from build123d import *
from build123d.topology import SkipClean

# Parameters (mm, degrees)
SKETCH1_R           = 8.89
BOSS_EXTRUDE1_DEPTH = 31.75
SKETCH2_R           = 3.302
BOSS_EXTRUDE2_DEPTH = 4.572
SKETCH3_R           = 11.938
BOSS_EXTRUDE3_DEPTH = 1.524


with BuildPart() as part:
    # Sketch1 → Boss-Extrude1 (new body)
    with BuildSketch(Plane(origin=(0, 0, 0), x_dir=(1, 0, 0), z_dir=(0, 1, 0))):
        with Locations(Location((0, 0, 0), (0, 0, 270))):
            Circle(SKETCH1_R)
    extrude(amount=BOSS_EXTRUDE1_DEPTH)

    # Sketch2 → Boss-Extrude2 (add)
    with BuildSketch(Plane(origin=(0, 31.75, 0), x_dir=(1, 0, 0), z_dir=(0, 1, 0))):
        with BuildLine():
            Line((2.607149425, 11.649833298), (23.651195402, 6.94032622))
            ThreePointArc((23.651195402, 6.94032622), (29.21, 0), (23.651195402, -6.94032622))
            Line((23.651195402, -6.94032622), (2.607149425, -11.649833298))
            ThreePointArc((2.607149425, -11.649833298), (-11.938, 0), (2.607149425, 11.649833298))
        make_face()
        with Locations(Location((22.098, 0, 0), (0, 0, 270))):
            Circle(SKETCH2_R, mode=Mode.SUBTRACT)
    extrude(amount=BOSS_EXTRUDE2_DEPTH)

    # Sketch3 → Boss-Extrude3 (add)
    with SkipClean():  # the faces are left unmerged after this step: merging them gives an invalid solid
        with BuildSketch(Plane(origin=(0, 36.322, 0), x_dir=(1, 0, 0), z_dir=(0, 1, 0))):
            with Locations(Location((0, 0, 0), (0, 0, 77.385465227))):
                Circle(SKETCH3_R)
        extrude(amount=BOSS_EXTRUDE3_DEPTH)


solid = part.part
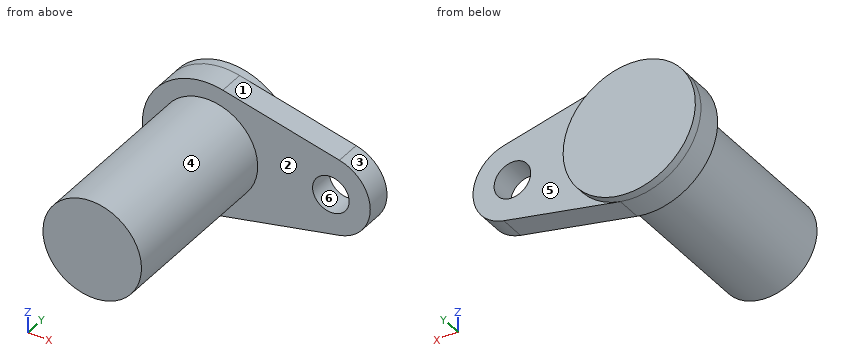
Design review of the part built by this model. Coordinates are the model's own, in mm. Face numbers are marked on the shaded views. A direction names the side the tool comes from. Round coordinates to 2 decimals unless told otherwise and drop trailing zeros. Write each loop counter-clockwise with the first axis right and the second up, starting at its lowest first coordinate (ties: lowest second). Pieces come first, ordered by that corner, then holes.
Item 1: For the marked faces 1 and 2, list the 3-axis set-ups (+Z, -Z, +X, -X, +Y, -Y) from which the entire face can be reached by the end or side of a thin tool; tool diameter is ignored.
Item 2: Consider section B-B on x = 0. Give the boundary of the cut face in (y, z).
Item 3: Consider section A-A on z = 0. Give the boundary of the cut face in (x, y).
Item 4: Consider section C-C on y = 29.5. Give the boundary of the cut face in (x, z), and give its area (3 significant figures).
Item 5: Consider section D-D on x = 11. Give the boundary of the cut face in (y, z), and give its area (3 significant figures).
Item 6: Draft analysis for pull direction X (two halves, no side actions). For the marked faces 3, 4, 5 and 6, state which applies: released by +X, released by -X, zero draft, split by the parting line, or undercut.
Item 7: Wall thickness on L1, parallel to X at y = 33.35, z = 0; L2, parallel to Y at x = 11.5, z = 4.5; L3, parallel to Y at x = 9.5, z = -1.25: over which ranges is each line inside the solid? List them lowest first.
Item 8: For pin 1 Ø1.5 at (x, y) = (8.5, 4.5) entering from +Z; pin 2 Ø5 at (x, z) = (20.5, -9) entering from +Y; pin 3 Ø5 at (x, y) = (4, 26.5) entering from +Z, all flat-tipped, find the tip position at first contact; note any pin that passes through.
Check values:
1. face 1: +Z, +X, +Y, -Y
1. face 2: -Y
2. outline: (0, -8.89) - (31.75, -8.89) - (31.75, -11.94) - (37.85, -11.94) - (37.85, 11.94) - (31.75, 11.94) - (31.75, 8.89) - (0, 8.89) - close
3. outline: (-11.94, 31.75) - (-8.89, 31.75) - (-8.89, 0) - (8.89, 0) - (8.89, 31.75) - (18.8, 31.75) - (18.8, 36.32) - (11.94, 36.32) - (11.94, 37.85) - (-11.94, 37.85) - close; (25.4, 31.75) - (29.21, 31.75) - (29.21, 36.32) - (25.4, 36.32) - close
4. outline: circle Ø17.78 at (0, 0)
4. area: 248 mm2
5. outline: (31.75, -9.77) - (36.32, -9.77) - (36.32, -4.64) - (37.85, -4.64) - (37.85, 4.64) - (36.32, 4.64) - (36.32, 9.77) - (31.75, 9.77) - close
5. area: 103 mm2
6. face 3: released by +X
6. face 4: split by the parting line
6. face 5: zero draft
6. face 6: undercut
7. L1: x = -11.94 to 18.8, 25.4 to 29.21
7. L2: y = 31.75 to 36.32
7. L3: y = 31.75 to 37.85
8. pin 1: stops at z = 4.36
8. pin 2: stops at y = 36.32
8. pin 3: stops at z = 8.76
